from build123d import *

# Parameters (mm, degrees)
F0_R     = 40
F0_R_2   = 38
F1_DEPTH = 180
F2_W     = 3
F2_H     = 90
F3_DEPTH = 160
F4_W     = 10
F4_H     = 50
F5_DEPTH = 66.8


with BuildPart() as f1:
    # F0 (on Top) → F1 (new body)
    with BuildSketch(Plane.XY):
        Circle(F0_R)
        Circle(F0_R_2, mode=Mode.SUBTRACT)
    extrude(amount=F1_DEPTH)

    # F2 (on Front) → F3 (cut)
    with BuildSketch(Plane.XZ):
        with Locations((0, 135)):
            Rectangle(F2_W, F2_H)
    extrude(amount=F3_DEPTH, mode=Mode.SUBTRACT)

    # F4 (on Front) → F5 (cut)
    with BuildSketch(Plane.XZ):
        with Locations((0, 25)):
            Rectangle(F4_W, F4_H)
    extrude(amount=-F5_DEPTH, mode=Mode.SUBTRACT)


solid = f1.part
The listing builds one solid part. Answer for the finished solid, in the listing's coordinates (mm). Coordinates: 2 decimals unless noted, no trailing zeros. Loops run counter-clockwise (first coordinate to the right, second up) from the corner with the lowest first, then second, coordinate; pieces in that order, holes last. Notation, with made-up numbers: (16.5, 65) -> (21.5, 65) arc R18 ccw to (21.5, 88) -> close; hole circle Ø9 at (-6.5, 41). An arc over 180 degrees is marked (long way). Answer in a Markdown table with one row per item. Add a question column.
1. The part is cut by section A-A, the plane y = 5.5. Write down the section's boundary in (x, z).
2. The part is cut by section D-D, the plane z = 123.5. Write down the section's boundary in (x, y), then the cut area to 3 significant figures.
3. Consider line 1 (X direction, y = 0, z = 40); line 2 (Y direction, x = -31, z = 170.5). Determine where each line is inside the solid, lowest interval first. Write a range as [from, to].
4. Flat-ended cylindrical pins translate along their axes: P1, Ø1, axis at x = 0.5, y = -39, coming from the +Z side; P2, Ø1, axis at x = 2.5, z = 78.5, coming from the +Y side; P3, Ø1.5, axis at y = 2, z = 53.5, coming from the -X side. Find the tip coordinate at first contact, or state that the pin passes through.
5. The part is cut by section C-C, the plane z = 59. Write down the section's boundary in (x, y).
6. The part is cut by section B-B, the plane x = -34. Write down the section's boundary in (y, z), then the cut area to 3 significant figures.
7. Determine the mould class of faces 1 (the cylindrical face through (-8.67, -39.05, 88.74)), 2 (the flat face through (35.4, -14.6, 180)), 3 (the cylindrical face through (-8.238, -37.096, 88.74)) for opening direction X: +X half, -X half, draft (parallel to the pull), parting line (faces both ways), or undercut.
Answer below:
| question | item | result |
|---|---|---|
| 1 | outline | (-39.62, 0) -> (-37.6, 0) -> (-37.6, 180) -> (-39.62, 180) -> close; (37.6, 0) -> (39.62, 0) -> (39.62, 180) -> (37.6, 180) -> close |
| 2 | outline | (-1.5, -39.97) -> (-1.5, -37.97) arc R38 cw (long way) to (1.5, -37.97) -> (1.5, -39.97) arc R40 ccw (long way) to start |
| 2 | area | 484 mm2 |
| 3 | line 1 | [-40, -38], [38, 40] |
| 3 | line 2 | [-25.28, -21.98], [21.98, 25.28] |
| 4 | P1 | z = 90 |
| 4 | P2 | y = 39.95 |
| 4 | P3 | x = -39.98 |
| 5 | outline | circle Ø80 at (0, 0); hole circle Ø76 at (0, 0) |
| 6 | outline | (-21.07, 0) -> (-16.97, 0) -> (-16.97, 180) -> (-21.07, 180) -> close; (16.97, 0) -> (21.07, 0) -> (21.07, 180) -> (16.97, 180) -> close |
| 6 | area | 1,480 mm2 |
| 7 | face 1 | parting line |
| 7 | face 2 | draft |
| 7 | face 3 | undercut |
